```python
from build123d import *

# Parameters (mm, degrees)
SKETCH_R  = 2.5
PAD_DEPTH = 50


with BuildPart() as part:
    # Sketch → Pad (new body)
    with BuildSketch(Plane.YZ):
        with BuildLine():
            ThreePointArc((-8, 10), (-9.414214, 9.414214), (-10, 8))
            Line((-10, 8), (-10, 3))
            Line((-8, 3), (-10, 3))
            Line((-8, 3), (-8, 7))
            Line((-4, 3), (-8, 7))
            Line((-4, -3), (-4, 3))
            Line((-8, -7), (-4, -3))
            Line((-8, -7), (-8, -3))
            Line((-10, -3), (-8, -3))
            Line((-10, -3), (-10, -8))
            ThreePointArc((-10, -8), (-9.414214, -9.414214), (-8, -10))
            Line((-8, -10), (-3, -10))
            Line((-3, -10), (-3, -8))
            Line((-3, -8), (-7, -8))
            Line((-3, -4), (-7, -8))
            Line((3, -4), (-3, -4))
            Line((3, -4), (7, -8))
            Line((3, -8), (7, -8))
            Line((3, -10), (3, -8))
            Line((3, -10), (8, -10))
            ThreePointArc((8, -10), (9.414214, -9.414214), (10, -8))
            Line((10, -8), (10, -3))
            Line((10, -3), (8, -3))
            Line((8, -7), (8, -3))
            Line((4, -3), (8, -7))
            Line((4, 3), (4, -3))
            Line((4, 3), (8, 7))
            Line((8, 7), (8, 3))
            Line((8, 3), (10, 3))
            Line((10, 3), (10, 8))
            ThreePointArc((10, 8), (9.414214, 9.414214), (8, 10))
            Line((3, 10), (8, 10))
            Line((3, 10), (3, 8))
            Line((3, 8), (7, 8))
            Line((7, 8), (3, 4))
            Line((-3, 4), (3, 4))
            Line((-3, 4), (-7, 8))
            Line((-7, 8), (-3, 8))
            Line((-3, 8), (-3, 10))
            Line((-8, 10), (-3, 10))
        make_face()
        Circle(SKETCH_R, mode=Mode.SUBTRACT)
    extrude(amount=PAD_DEPTH)


solid = part.part
```
Could you check a few things on this model? Use its own coordinates, in mm. A direction names the side the tool comes from. Coordinates: 2 decimals unless noted, no trailing zeros. Write each loop counter-clockwise with the first axis right and the second up, starting at its lowest first coordinate (ties: lowest second). Pieces come first, ordered by that corner, then holes. Notation, with made-up numbers: M 61.25,-37 L 95.25,-37 A22 ccw 95.25,-29 Z; hole C 45.25,47.25 d3. An arc over 180 degrees is marked long. Answer as CSV lines item,"result". Start each with the question number.
1) We'd pull the mould along Y, two halves only. Please class faces 1 (the flat face through (25, -5, -6)), 2 (the flat face through (25, -10, -5)), 3 (the flat face through (25, 4, 0)): +Y half, -Y half, draft (parallel to the pull), parting line (faces both ways), or undercut.
2) I want a section at A-A, the plane z = -5.75. Please give me the cut outline in (x, y), and give its area (3 significant figures).
3) For P1, Ø1.6, axis at x = 35, z = -9.5, coming from the +Y side; P2, Ø6, axis at y = 0, z = 0, coming from the +X side; P3, Ø0.6, axis at x = 37, y = 9, coming from the -Z side; P4, Ø0.6, axis at x = 37, z = 8.5, coming from the -Y side, each with a flat end and sliding along its axis, tell me the tip position at first contact or that it passes through.
4) I want a section at B-B, the plane y = 0. Please give me the cut outline in (x, z).
5) Please list where these lines run through material, in increasing order: line 1 (Z direction, x = 19.5, y = 0); line 2 (Z direction, x = 16, y = -4.5); line 3 (Y direction, x = 19.5, z = 6.5). Write a range as from..to.
6) I want a section at D-D, the plane y = 3.5. Please give me the cut outline in (x, z), and give its area (3 significant figures).
7) For faces 4 (the flat face through (25, -6, -5)), 5 (the flat face through (25, -3, -9)), 6 (the flat face through (25, 9, 3)), 7 (the flat face through (25, 0, 4)), which set-ups out of +Z, -Z, +X, -X, +Y, -Y let a thin tool reach every point of the face, with its end or its side?
Data:
1,face 1,"undercut"
1,face 2,"-Y half"
1,face 3,"+Y half"
2,outline,"M 0,-10 L 50,-10 L 50,-8 L 0,-8 Z; M 0,-6.75 L 50,-6.75 L 50,-4.75 L 0,-4.75 Z; M 0,4.75 L 50,4.75 L 50,6.75 L 0,6.75 Z; M 0,8 L 50,8 L 50,10 L 0,10 Z"
2,area,"400 mm^2"
3,P1,"stops at y = 9.87"
3,P2,"stops at x = 50"
3,P3,"stops at z = -9.87"
3,P4,"stops at y = -9.99"
4,outline,"M 0,-4 L 50,-4 L 50,-2.5 L 0,-2.5 Z; M 0,2.5 L 50,2.5 L 50,4 L 0,4 Z"
5,line 1,"z = -4..-2.5, 2.5..4"
5,line 2,"z = -10..-8, -5.5..-3.5, 3.5..5.5, 8..10"
5,line 3,"y = -10..-8, -7.5..-5.5, 5.5..7.5, 8..10"
6,outline,"M 0,-10 L 50,-10 L 50,-8 L 0,-8 Z; M 0,-4.5 L 50,-4.5 L 50,4.5 L 0,4.5 Z; M 0,8 L 50,8 L 50,10 L 0,10 Z"
6,area,"650 mm^2"
7,face 4,"+X, -X"
7,face 5,"-Z, +X, -X"
7,face 6,"+X, -X, +Y"
7,face 7,"+Z, +X, -X"
